Check sheet for the modelled part. Datum: model origin and axes. Units: mm. Give positions to 0.01 mm unless a question says otherwise; leave off trailing zeros. Order: outer loops, then holes, each group sorted by start corner. A loop starts at its lowest first (then second) coordinate and runs counter-clockwise, first axis right, second up.
Item 1: Sectioned sample at B-B on z = 0. Record the boundary of the cut face in (x, y), and give its area (3 significant figures).
Item 2: Sectioned sample at A-A on y = 0. Record the boundary of the cut face in (x, z).
Item 3: Material ranges on line 1 along Z through (x, y) = (2.7, 0); line 2 along Y through (x, z) = (3.6, 1); line 3 along Y through (x, z) = (2.2, 1.25), recorded low to high.
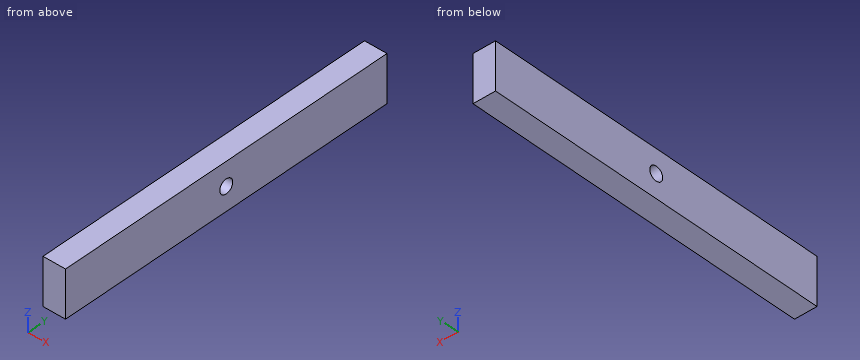
Autodesk Fusion 360 part; units mm, degrees
sketch "Sketch1" plane through (0, 0, 0) normal (1, 0, 0) x (0, 1, 0)
  line L0 (-37.3, 5) -> (37.3, 5)
  line L1 (37.3, 5) -> (37.3, -5)
  line L2 (37.3, -5) -> (-37.3, -5)
  line L3 (-37.3, -5) -> (-37.3, 5)
  line L4 (0, 0) -> (0, 5) construction
  line L5 (0, 0) -> (-37.3, 0) construction
  circle A0 centre (0, 0) radius 1.5
  point P0 (0, 5)
  point P1 (-37.3, 0)
  dimension "d1" = 3
  dimension "d2" = 10
  dimension "d3" = 74.6
extrude "Extrude1" add sketch "Sketch1" along normal blind 4.8
Report:
1. outline: (0, -37.3) - (4.8, -37.3) - (4.8, -1.5) - (0, -1.5) - close; (0, 1.5) - (4.8, 1.5) - (4.8, 37.3) - (0, 37.3) - close
1. area: 344 mm2
2. outline: (0, -5) - (4.8, -5) - (4.8, -1.5) - (0, -1.5) - close; (0, 1.5) - (4.8, 1.5) - (4.8, 5) - (0, 5) - close
3. line 1: z = -5 to -1.5, 1.5 to 5
3. line 2: y = -37.3 to -1.12, 1.12 to 37.3
3. line 3: y = -37.3 to -0.83, 0.83 to 37.3
